The listing builds one solid part. Answer for the finished solid, in the listing's coordinates (mm). Give positions to 0.01 mm unless a question says otherwise; leave off trailing zeros. Loops run counter-clockwise (first coordinate to the right, second up) from the corner with the lowest first, then second, coordinate; pieces in that order, holes last. Notation, with made-up numbers: M 25.5,47.5 L 63.5,47.5 A29 ccw 63.5,85.5 Z; hole C 85.25,48.5 d4. An arc over 180 degrees is marked long. Return JSON: item names as keys, results as strings.
from build123d import *

# Parameters (mm, degrees)
F0_R     = 18.1237353156
F0_R_2   = 14.9714122035
F0_R_3   = 12.3128911041
F0_R_4   = 10.0708194052
F0_R_5   = 8.1799615502
F0_R_6   = 6.5853009382
F0_R_7   = 5.2404391544
F0_R_8   = 4
F1_DEPTH = 5
F2_R     = 2.49999


# Not quite as in the source:
# - a fillet or chamfer is up to 0.001 mm smaller than in the source, because OpenCascade refuses the exact size


with BuildPart() as f1:
    # F0 (on Front) → F1 (new body)
    with BuildSketch(Plane.XZ):
        with BuildLine():
            ThreePointArc((3.1164704126, -2.5075111501), (-1.3293077803, -3.7726569981), (-4, 0))
            Line((-4, 0), (-4, 5))
            Line((-4, 5), (-9, 5))
            Line((-9, 5), (-9, 0))
            ThreePointArc((-9, 0), (-7.9372539332, -4.2426406871), (-5, -7.4833147735))
            Line((-5, -7.4833147735), (-5, -16))
            Line((-5, -16), (0, -16))
            ThreePointArc((0, -16), (2.8284271247, -17.1715728753), (4, -20))
            ThreePointArc((4, -20), (3.4641016151, -22), (2, -23.4641016151))
            Line((2, -23.4641016151), (-9.3205080757, -30))
            Line((-9.3205080757, -30), (40.2062176005, -30))
            Line((40.2062176005, -30), (126.9921824081, 126.1129207402))
            ThreePointArc((126.9921824081, 126.1129207402), (124.4672099784, 136.6365680143), (113.7670591749, 135.0150223001))
            Line((113.7670591749, 135.0150223001), (3.1164704126, -2.5075111501))
        make_face()
        with Locations((27.1926598128, -7.8762646844)):
            Circle(F0_R, mode=Mode.SUBTRACT)
        with Locations((47.9066364562, 22.8967940046)):
            Circle(F0_R_2, mode=Mode.SUBTRACT)
        with Locations((65.375830444, 48.8493448398)):
            Circle(F0_R_3, mode=Mode.SUBTRACT)
        with Locations((80.1085273008, 70.736505998)):
            Circle(F0_R_4, mode=Mode.SUBTRACT)
        with Locations((92.5333911397, 89.1951086458)):
            Circle(F0_R_5, mode=Mode.SUBTRACT)
        with Locations((103.0119371191, 104.7622262472)):
            Circle(F0_R_6, mode=Mode.SUBTRACT)
        with Locations((111.8490501262, 117.8908013099)):
            Circle(F0_R_7, mode=Mode.SUBTRACT)
        with Locations((120, 130)):
            Circle(F0_R_8, mode=Mode.SUBTRACT)
    extrude(amount=F1_DEPTH)

    # F2 (radius 2.5 in the source; OpenCascade refuses exactly that, so slightly less here)
    f2_edges = [f1.edges().sort_by_distance(p)[0] for p in [
        (-9, -2.5, 5),
        (-4, -2.5, 5),
        (-9.320508, -2.5, -30),
        (40.206218, -2.5, -30),
        (-5, -2.5, -7.483315),
        (-5, -2.5, -16),
    ]]
    fillet(f2_edges, radius=F2_R)


solid = f1.part
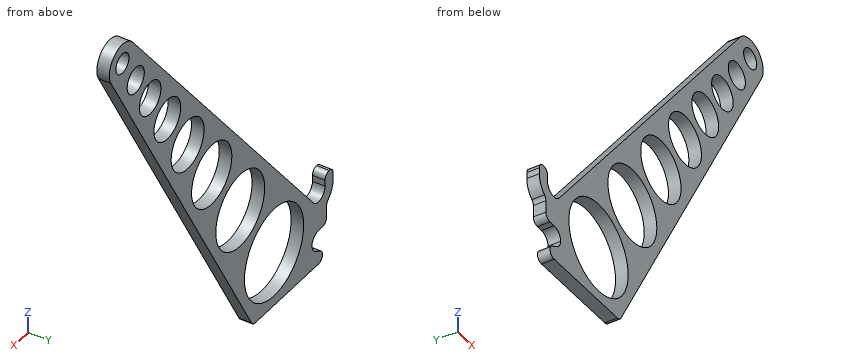
(1) Given pin 1 (0.8 mm diameter, centred on x = -2, y = -2, fed in from -Z); pin 2 (1.3 mm diameter, centred on y = -3, z = 1.5, fed in from +X); pin 3 (1 mm diameter, centred on x = 37.5, y = -3.5, fed in from +Z); pin 4 (18 mm diameter, centred on x = 80.11, z = 70.74, fed in from -Y), each flat-ended and moving along its own axis, determine where each tip first touches the part or whether it passes through.
Values follow:
{"pin 1": "z = -29.41", "pin 2": "x = 58.08", "pin 3": "z = 40.85", "pin 4": "through"}
(2) The part is cut by section C-C (y = -2.25). Give the number of separate pieces and of enclosed holes in the cut face, and give its area (3 significant figures).
Values follow:
{"separate pieces": "1", "enclosed holes": "8", "area": "3,250 mm²"}
(3) The part is cut by section A-A (x = 21). Determine the outline of the cut face in (y, z).
Values follow:
{"outline": "M -5,-30 L 0,-30 L 0,-24.91 L -5,-24.91 Z; M -5,9.16 L 0,9.16 L 0,19.72 L -5,19.72 Z"}
(4) The part is cut by section B-B (z = 130). Determine the outline of the cut face in (x, y).
Values follow:
{"outline": "M 109.73,-5 L 116,-5 L 116,0 L 109.73,0 Z; M 124,-5 L 128,-5 L 128,0 L 124,0 Z"}
(5) Straight lines are drawn through the part: line 1 along Z through (x, y) = (108, -2.5); line 2 along X through (y, z) = (-0.6, -15); line 3 along X through (y, z) = (-2.4, 28.5). For each, find the intervals that lie inside material, in ascending order.
Values follow:
{"line 1": "91.95 to 100.46, 109.06 to 114.33, 121.45 to 127.85", "line 2": "-4.5 to 10.53, 43.86 to 48.54", "line 3": "28.07 to 34.02, 61.79 to 72.73"}
